```python
from build123d import *

# Parameters (mm, degrees)
SKETCH4_W           = 106
SKETCH4_H           = 106
BOSS_EXTRUDE3_DEPTH = 5
SKETCH6_W           = 101
SKETCH6_H           = 101
CUT_EXTRUDE2_DEPTH  = 3
SKETCH7_R           = 3.5
BOSS_EXTRUDE4_DEPTH = 3
FILLET1_R           = 3
SKETCH10_W          = 103
SKETCH10_H          = 103
SKETCH10_W_2        = 101
SKETCH10_H_2        = 101
BOSS_EXTRUDE5_DEPTH = 2


with BuildPart() as part:
    # Sketch4 → Boss-Extrude3 (new body)
    with BuildSketch(Plane(origin=(0, 0, 0), x_dir=(1, 0, 0), z_dir=(0, 1, 0))):
        with Locations((-47.689542484, -44.460784314)):
            Rectangle(SKETCH4_W, SKETCH4_H)
    extrude(amount=BOSS_EXTRUDE3_DEPTH)

    # Sketch6 → Cut-Extrude2 (cut)
    with BuildSketch(Plane(origin=(0, 5, 0), x_dir=(1, 0, 0), z_dir=(0, 1, 0))):
        with Locations((-47.689542484, -44.460784314)):
            Rectangle(SKETCH6_W, SKETCH6_H)
    extrude(amount=-CUT_EXTRUDE2_DEPTH, mode=Mode.SUBTRACT)

    # Sketch7 → Boss-Extrude4 (add)
    with BuildSketch(Plane(origin=(0, 2, 0), x_dir=(1, 0, 0), z_dir=(0, 1, 0))):
        with Locations(Location((-92.689542484, -24.610784314, 0), (0, 0, 270))):
            Circle(SKETCH7_R)
        with Locations(Location((-92.689542484, -89.460784314, 0), (0, 0, 270))):
            Circle(SKETCH7_R)
        with Locations(Location((-2.689542484, -89.460784314, 0), (0, 0, 270))):
            Circle(SKETCH7_R)
        with Locations(Location((-2.689542484, -24.610784314, 0), (0, 0, 270))):
            Circle(SKETCH7_R)
    extrude(amount=BOSS_EXTRUDE4_DEPTH)

    # Fillet1
    fillet1_edges = [part.edges().sort_by_distance(p)[0] for p in [
        (-47.689542484, 0, 97.460784314),
        (-100.689542484, 0, 44.460784314),
        (-47.689542484, 0, -8.539215686),
        (5.310457516, 0, 44.460784314),
    ]]
    fillet(fillet1_edges, radius=FILLET1_R)

    # Sketch10 → Boss-Extrude5 (add)
    with BuildSketch(Plane(origin=(0, 5, 0), x_dir=(1, 0, 0), z_dir=(0, 1, 0))):
        with Locations((-47.689542484, -44.460784314)):
            Rectangle(SKETCH10_W, SKETCH10_H)
        with Locations((-47.689542484, -44.460784314)):
            Rectangle(SKETCH10_W_2, SKETCH10_H_2, mode=Mode.SUBTRACT)
    extrude(amount=BOSS_EXTRUDE5_DEPTH)


solid = part.part
```
Part model, mm, in its own coordinate system. A direction names the side the tool comes from. Round coordinates to 2 decimals unless told otherwise and drop trailing zeros. Order: outer loops, then holes, each group sorted by start corner. A loop starts at its lowest first (then second) coordinate and runs counter-clockwise, first axis right, second up. Notation, with made-up numbers: M -4,-6.5 L 14,-6.5 A27 cw 14,15.5 Z; hole C -12,28.5 d5. An arc over 180 degrees is marked long. Answer in a Markdown table with one row per item. Add a question column.
Q1. Mould opens along X. For faces 3 (the face through (-46.95, 0.9, -7.68)), 4 (the face through (-99.83, 0.9, 43.72)), 5 (the face through (-3, 5, 25)) say: +X half, -X half, draft (parallel to the pull), parting line (faces both ways), or undercut.
Q2. Wall check: L1, parallel to X at y = 3.5, z = 77; L2, parallel to Z at x = -40.5, y = 6.75; L3, parallel to Z at x = -85.5, y = 3.75. Give the ranges that are in metal, low to high. Write a range as from..to.
Q3. Cut at B-B on x = -23.5. Give the cut face in (y, z), and give its area (3 significant figures).
Q4. Cut at C-C on z = 91. Give the cut face in (x, y), and give its area (3 significant figures).
Q5. 3-axis set-ups, long thin cutter, end or side, ignore diameter. For faces 1 (the face through (4.408, 0.855, 43.719)), 2 (the face through (-93, 5, 89)): which of +Z, -Z, +X, -X, +Y, -Y reach the whole face in a straight line?
Q6. Pin check, flat tips, straight feed: pin 1 (1.6 mm diameter, centred on y = 6, z = 58.5, fed in from -X); pin 2 (1 mm diameter, centred on x = -33.5, y = 6, fed in from +Z); pin 3 (4 mm diameter, centred on y = 5.5, z = 42.5, fed in from +X); pin 4 (7.5 mm diameter, centred on x = -4, z = 26.5, fed in from +Y). Stop position of each tip, or through.
Q7. Cut at A-A on z = 74. Give the cut face in (x, y), and give its area (3 significant figures).
Established:
| question | item | result |
|---|---|---|
| 1 | face 3 | draft |
| 1 | face 4 | -X half |
| 1 | face 5 | undercut |
| 2 | L1 | x = -100.69..-98.19, 2.81..5.31 |
| 2 | L2 | z = -7.04..-6.04, 94.96..95.96 |
| 2 | L3 | z = -8.54..-6.04, 94.96..97.46 |
| 3 | outline | M 0,-5.54 A3 ccw 3,-8.54 L 5,-8.54 L 5,-7.04 L 7,-7.04 L 7,-6.04 L 2,-6.04 L 2,94.96 L 7,94.96 L 7,95.96 L 5,95.96 L 5,97.46 L 3,97.46 A3 ccw 0,94.46 Z |
| 3 | area | 227 mm2 |
| 4 | outline | M -100.69,3 A3 ccw -97.69,0 L 2.31,0 A3 ccw 5.31,3 L 5.31,5 L 3.81,5 L 3.81,7 L 2.81,7 L 2.81,2 L 0.45,2 L 0.45,5 L -5.83,5 L -5.83,2 L -89.55,2 L -89.55,5 L -95.83,5 L -95.83,2 L -98.19,2 L -98.19,7 L -99.19,7 L -99.19,5 L -100.69,5 Z |
| 4 | area | 265 mm2 |
| 5 | face 1 | +Z, -Z, +X, -Y |
| 5 | face 2 | +Y |
| 6 | pin 1 | stops at x = -99.19 |
| 6 | pin 2 | stops at z = 95.96 |
| 6 | pin 3 | stops at x = 5.31 |
| 6 | pin 4 | stops at y = 5 |
| 7 | outline | M -100.69,3 A3 ccw -97.69,0 L 2.31,0 A3 ccw 5.31,3 L 5.31,5 L 3.81,5 L 3.81,7 L 2.81,7 L 2.81,2 L -98.19,2 L -98.19,7 L -99.19,7 L -99.19,5 L -100.69,5 Z |
| 7 | area | 227 mm2 |
